Can you work these out from the model? Positions are in its coordinate system, mm. A direction names the side the tool comes from. Round coordinates to 2 decimals unless told otherwise and drop trailing zeros. Loops run counter-clockwise (first coordinate to the right, second up) from the corner with the lowest first, then second, coordinate; pieces in that order, holes last. Notation, with made-up numbers: (-37, 76) -> (6, 76) arc R22 ccw to (6, 89) -> close; hole circle Ø2 at (64.25, 87.5). An arc over 180 degrees is marked (long way). Use a Markdown table: item, result.
from build123d import *

# Parameters (mm, degrees)
SKETCH1_W                   = 76.2
SKETCH1_H                   = 63.5
BOSS_EXTRUDE1_DEPTH         = 19.05
SKETCH2_W                   = 55.88
SKETCH2_H                   = 63.5
CUT_EXTRUDE1_DEPTH          = 13.97
F_1_4_20_TAPPED_HOLE1_D     = 5.1054
F_1_4_20_TAPPED_HOLE1_DEPTH = 19.05
F_1_4_20_TAPPED_HOLE1_TIP   = 1.533816902
LPATTERN1_COUNT             = 2
LPATTERN1_PITCH             = 57.15
LPATTERN1_COUNT_DIR2        = 2
LPATTERN1_PITCH_DIR2        = 63.5
SKETCH7_W                   = 76.2
SKETCH7_H                   = 38.1
CUT_EXTRUDE2_DEPTH          = 13.97


with BuildPart() as part:
    # Sketch1 → Boss-Extrude1 (new body)
    with BuildSketch(Plane(origin=(0, 0, 0), x_dir=(0, 0, -1), z_dir=(1, 0, 0))):
        Rectangle(SKETCH1_W, SKETCH1_H)
    extrude(amount=BOSS_EXTRUDE1_DEPTH)

    # Sketch2 → Cut-Extrude1 (cut)
    with BuildSketch(Plane(origin=(19.05, 0, 0), x_dir=(0, 0, -1), z_dir=(1, 0, 0))):
        Rectangle(SKETCH2_W, SKETCH2_H)
    extrude(amount=-CUT_EXTRUDE1_DEPTH, mode=Mode.SUBTRACT)

    # Sketch5 → #10-32 Tapped Hole1 (revolve, cut)
    with BuildSketch(Plane(origin=(19.05, 28.575, 31.75), x_dir=(0, 0, -1), z_dir=(0, 1, 0))):
        Polygon((0, 0), (0, 14.929317848), (2.0193, 13.716), (2.0193, 0), align=None)
    f_10_32_tapped_hole1 = revolve(axis=Axis((25.4, 28.575, 31.75), (-1, 0, 0)), mode=Mode.SUBTRACT)

    # 1/4-20 Tapped Hole1
    with Locations(Plane(origin=(5.08, 0, 0), x_dir=(0, 0, -1), z_dir=(1, 0, 0))):
        with Locations((0, 9.525)):
            Hole(F_1_4_20_TAPPED_HOLE1_D / 2, depth=F_1_4_20_TAPPED_HOLE1_DEPTH)
            with Locations((0, 0, -(F_1_4_20_TAPPED_HOLE1_DEPTH + F_1_4_20_TAPPED_HOLE1_TIP / 2))):  # 118° drill point
                Cone(0, F_1_4_20_TAPPED_HOLE1_D / 2, F_1_4_20_TAPPED_HOLE1_TIP, mode=Mode.SUBTRACT)

    # LPattern1: 10-32 Tapped Hole1 2 × 2
    with Locations(*[(0, -i * LPATTERN1_PITCH, -j * LPATTERN1_PITCH_DIR2) for i in range(LPATTERN1_COUNT) for j in range(LPATTERN1_COUNT_DIR2) if (i, j) != (0, 0)]):
        add(f_10_32_tapped_hole1, mode=Mode.SUBTRACT)

    # Sketch7 → Cut-Extrude2 (cut)
    with BuildSketch(Plane(origin=(19.05, 0, 0), x_dir=(0, 0, -1), z_dir=(1, 0, 0))):
        Rectangle(SKETCH7_W, SKETCH7_H)
    extrude(amount=-CUT_EXTRUDE2_DEPTH, mode=Mode.SUBTRACT)


solid = part.part
1. I want a section at B-B (z = 0). Please give me the cut outline in (x, y), plus the area to 3 significant figures.
Answer sheet:
| item | result |
|---|---|
| outline | (0, -31.75) -> (5.08, -31.75) -> (5.08, 6.97) -> (0, 6.97) -> close; (0, 12.08) -> (5.08, 12.08) -> (5.08, 31.75) -> (0, 31.75) -> close |
| area | 297 mm² |
2. Which directions (+Z, -Z, +X, -X, +Y, -Y) give clear straight access to the entire face, cutting with the end or side of a thin tool? Please do faces 1 (the flat face through (12, -25, 27.94)), 2 (the cylindrical face through (2.504, 7.033, -0.553)), 3 (the cylindrical face through (12.288, 27.968, -33.676)), 4 (the flat face through (12, 19.05, 33)), 5 (the flat face through (19.05, 25, 33)).
Answer sheet:
| item | result |
|---|---|
| face 1 | +X, +Y, -Y |
| face 2 | +X, -X |
| face 3 | +X |
| face 4 | +Z, -Z, +X |
| face 5 | +Z, -Z, +X, +Y, -Y |
3. I want a section at C-C (y = -20). Please give me the cut outline in (x, z).
Answer sheet:
| item | result |
|---|---|
| outline | (0, -38.1) -> (19.05, -38.1) -> (19.05, -27.94) -> (5.08, -27.94) -> (5.08, 27.94) -> (19.05, 27.94) -> (19.05, 38.1) -> (0, 38.1) -> close |
4. If we mould it in two halves opening along Z, with no side actions, what happens to faces 6 (the flat face through (19.05, 25, -33)), 7 (the flat face through (12, -25, -27.94)), 8 (the flat face through (3, 0, 38.1)), 9 (the conical face through (4.331, 28.886, -31.912))? For each: +Z half, -Z half, draft (parallel to the pull), parting line (faces both ways), or undercut.
Answer sheet:
| item | result |
|---|---|
| face 6 | draft |
| face 7 | undercut |
| face 8 | +Z half |
| face 9 | undercut |
5. I want a section at A-A (x = 14.5). Please give me the cut outline in (y, z) (3 decimals).
Answer sheet:
| item | result |
|---|---|
| outline | (-31.75, -38.1) -> (-19.05, -38.1) -> (-19.05, -27.94) -> (-31.75, -27.94) -> close; (-31.75, 27.94) -> (-19.05, 27.94) -> (-19.05, 38.1) -> (-31.75, 38.1) -> close; (19.05, -38.1) -> (31.75, -38.1) -> (31.75, -27.94) -> (19.05, -27.94) -> close; (19.05, 27.94) -> (31.75, 27.94) -> (31.75, 38.1) -> (19.05, 38.1) -> close; hole circle Ø4.039 at (-28.575, -31.75); hole circle Ø4.039 at (-28.575, 31.75); hole circle Ø4.039 at (28.575, -31.75); hole circle Ø4.039 at (28.575, 31.75) |
6. Will these pins go through, and if not, where does the flat tip stop? pin 1 Ø3 at (y, z) = (9.525, 0) entering from -X; pin 2 Ø3.5 at (y, z) = (28.575, 31.75) entering from +X.
Answer sheet:
| item | result |
|---|---|
| pin 1 | passes through |
| pin 2 | stops at x = 5.17 |
7. I need wall thicknesses on line 1 (Y direction, x = 10, z = 31.75); line 2 (Z direction, x = 10.5, y = 21.5); line 3 (Y direction, x = 1.65, z = 0). Which ranges of each line are inside material? Lowest first, please.
Answer sheet:
| item | result |
|---|---|
| line 1 | y = -31.75 to -30.59, -26.56 to -19.05, 19.05 to 26.56, 30.59 to 31.75 |
| line 2 | z = -38.1 to -27.94, 27.94 to 38.1 |
| line 3 | y = -31.75 to 6.97, 12.08 to 31.75 |
